from build123d import *

# Parameters (mm, degrees)
PAD_DEPTH    = 24
SKETCH002_R  = 7.732913
PAD001_DEPTH = 20
SKETCH001_W  = 6
SKETCH001_H  = 14
POCKET_DEPTH = 11


with BuildPart() as part:
    # Sketch → Pad (new body)
    with BuildSketch(Plane.XZ):
        Polygon((-9.577921, 39.93367), (-30, 39.93367), (-30, 28.000008), (-20, 28.000008), (-20, 2.029604), (-30, 2.029604), (-30, -2), (-9.99258, -2), (-9.99258, -10), (-40, -10), (-40, 50.000008), (-9.577921, 50.000008), align=None)
    extrude(amount=PAD_DEPTH)

    # Sketch002 → Pad001 (join)
    with BuildSketch(Plane(origin=(-40, 0, 0), x_dir=(0, 0, -1), z_dir=(-1, 0, 0))):
        with Locations((-20, 12)):
            Circle(SKETCH002_R)
    extrude(amount=PAD001_DEPTH)

    # Sketch001 (on Face11 of Pad) → Pocket (cut)
    with BuildSketch(Plane(origin=(0, 0, 50.000008), x_dir=(-1, 0, 0), z_dir=(0, 0, 1))):
        with Locations((26, 12.048018)):
            Rectangle(SKETCH001_W, SKETCH001_H)
    extrude(amount=-POCKET_DEPTH, mode=Mode.SUBTRACT)


solid = part.part
CAD build for the part. Positions are in the model's coordinates, mm. A direction names the side the tool comes from. Coordinates: 2 decimals unless noted, no trailing zeros. Write each loop counter-clockwise with the first axis right and the second up, starting at its lowest first coordinate (ties: lowest second). Pieces come first, ordered by that corner, then holes. Notation, with made-up numbers: (-24.75, -33) - (-19.75, -33) arc R16 cw to (-19.75, -23) - close; hole circle Ø2 at (-20.5, 76). An arc over 180 degrees is marked (long way). Use a Markdown table: item, result. Add a question column.
Item 1: Band-saw the part on D-D, the plane z = 41. Give the cut face in (x, y), and give its area (3 significant figures).
Item 2: Band-saw the part on B-B, the plane z = 20. Give the cut face in (x, y), and give its area (3 significant figures).
Item 3: Band-saw the part on A-A, the plane y = -12. Give the cut face in (x, z).
Item 4: Band-saw the part on C-C, the plane x = -16. Give the cut face in (y, z), and give its area (3 significant figures).
Item 5: Flat gauge pins, fed straight in: pin 1 (7 mm diameter, centred on y = -16.5, z = 10, fed in from +X); pin 2 (6 mm diameter, centred on y = -14, z = 35.5, fed in from +X); pin 3 (6 mm diameter, centred on x = -53.5, z = 14.5, fed in from -Y). Where does each tip first touch, or does it go through?
Item 6: Drill centre lines: L1, parallel to Z at x = -29, y = -2; L2, parallel to Z at x = -15.5, y = -14; L3, parallel to X at y = -21.25, z = 25. Where is each one in solid material? Low to high. Write a range as from..to.
Item 7: Mould opens along Z. For faces 5 (the face through (-25, -12, 28)), 6 (the face through (-60, -12, 20)), 7 (the face through (-22, -12, 50)) say: pulls with the +Z half, pulls with the -Z half, needs draft (parallel to the pull), parting line crosses it, or undercut.
Item 8: 3-axis set-ups, long thin cutter, end or side, ignore diameter. For faces 1 (the face through (-49.86, -9.038, 12.857)), 2 (the face through (-23, -12, 45)), 3 (the face through (-17, -12, 39.934)), 4 (the face through (-9.993, -12, -6)): which of +Z, -Z, +X, -X, +Y, -Y reach the whole face in a straight line?
Numbers:
| question | item | result |
|---|---|---|
| 1 | outline | (-40, -24) - (-9.58, -24) - (-9.58, 0) - (-40, 0) - close; hole (-29, -19.05) - (-23, -19.05) - (-23, -5.05) - (-29, -5.05) - close |
| 1 | area | 646 mm2 |
| 2 | outline | (-60, -19.73) - (-40, -19.73) - (-40, -24) - (-20, -24) - (-20, 0) - (-40, 0) - (-40, -4.27) - (-60, -4.27) - close |
| 2 | area | 789 mm2 |
| 3 | outline | (-60, 12.27) - (-40, 12.27) - (-40, -10) - (-9.99, -10) - (-9.99, -2) - (-30, -2) - (-30, 2.03) - (-20, 2.03) - (-20, 28) - (-30, 28) - (-30, 39.93) - (-29, 39.93) - (-29, 50) - (-40, 50) - (-40, 27.73) - (-60, 27.73) - close; (-23, 39.93) - (-9.58, 39.93) - (-9.58, 50) - (-23, 50) - close |
| 4 | outline | (-24, -10) - (0, -10) - (0, -2) - (-24, -2) - close; (-24, 39.93) - (0, 39.93) - (0, 50) - (-24, 50) - close |
| 4 | area | 434 mm2 |
| 5 | pin 1 | x = -20 |
| 5 | pin 2 | x = -30 |
| 5 | pin 3 | y = -19.32 |
| 6 | L1 | -10..-2, 2.03..28, 39.93..50 |
| 6 | L2 | -10..-2, 39.93..50 |
| 6 | L3 | -40..-20 |
| 7 | face 5 | undercut |
| 7 | face 6 | needs draft |
| 7 | face 7 | pulls with the +Z half |
| 8 | face 1 | -X |
| 8 | face 2 | +Z |
| 8 | face 3 | +X, +Y, -Y |
| 8 | face 4 | -Z, +X, +Y, -Y |
